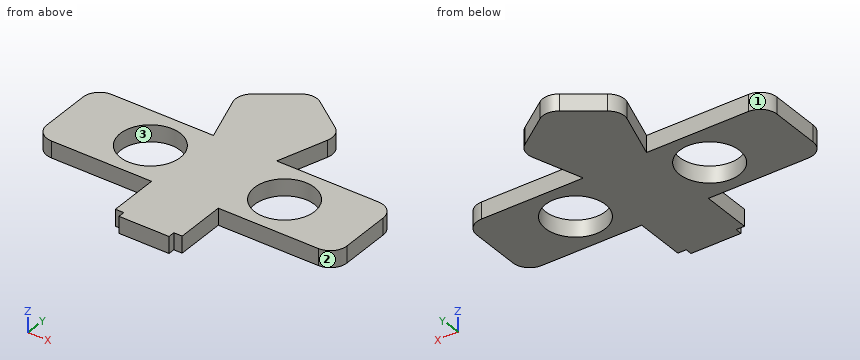
from build123d import *

# Parameters (mm, degrees)
F0_R     = 9
F0_W     = 15
F0_H     = 2
F1_DEPTH = 5


with BuildPart() as f1:
    # F0 (on Top) → F1 (new body)
    with BuildSketch(Plane.XY):
        with BuildLine():
            Line((-9.487151, 12.5), (-40, 12.5))
            ThreePointArc((-40, 12.5), (-43.535534, 11.035534), (-45, 7.5))
            Line((-45, 7.5), (-45, -7.5))
            ThreePointArc((-45, -7.5), (-43.535534, -11.035534), (-40, -12.5))
            Line((-40, -12.5), (-10, -12.5))
            Line((-10, -12.5), (10, -12.5))
            Line((10, -12.5), (40, -12.5))
            ThreePointArc((40, -12.5), (43.535534, -11.035534), (45, -7.5))
            Line((45, -7.5), (45, 7.5))
            ThreePointArc((45, 7.5), (43.535534, 11.035534), (40, 12.5))
            Line((40, 12.5), (9.487151, 12.5))
            Line((9.487151, 12.5), (-9.487151, 12.5))
        make_face()
        with Locations((-19.38206, 0)):
            Circle(F0_R, mode=Mode.SUBTRACT)
        with Locations((20.852027, 0)):
            Circle(F0_R, mode=Mode.SUBTRACT)
        with BuildLine():
            Line((-14.227962, 27.090718), (-9.487151, 12.5))
            Line((-9.487151, 12.5), (9.487151, 12.5))
            Line((9.487151, 12.5), (14.227962, 27.090718))
            ThreePointArc((14.227962, 27.090718), (14.227962, 30.180888), (12.411606, 32.680888))
            Line((12.411606, 32.680888), (2.938926, 39.563193))
            ThreePointArc((2.938926, 39.563193), (0, 40.518108), (-2.938926, 39.563193))
            Line((-2.938926, 39.563193), (-12.411606, 32.680888))
            ThreePointArc((-12.411606, 32.680888), (-14.227962, 30.180888), (-14.227962, 27.090718))
        make_face()
        Polygon((10, -12.5), (-10, -12.5), (-10, -27.5), (-7.5, -27.5), (7.5, -27.5), (10, -27.5), align=None)
        with Locations((0, -28.5)):
            Rectangle(F0_W, F0_H)
    extrude(amount=F1_DEPTH)


solid = f1.part
The model under review builds one solid part; all positions refer to its coordinate system, in mm. Face numbers are marked on the shaded views. Coordinates: 2 decimals unless noted, no trailing zeros. Write each loop counter-clockwise with the first axis right and the second up, starting at its lowest first coordinate (ties: lowest second). Pieces come first, ordered by that corner, then holes. Notation, with made-up numbers: (-27.75, 71.5) - (0.25, 71.5) arc R23 ccw to (0.25, 92.5) - close; hole circle Ø5 at (-30.75, 39). An arc over 180 degrees is marked (long way). Answer as CSV lines item,"result".
(1) We need section A-A (y = 0). Give the boundary of the cut face in (x, z), plus the area to 3 significant figures.
Data:
outline,"(-45, 0) - (-28.38, 0) - (-28.38, 5) - (-45, 5) - close; (-10.38, 0) - (11.85, 0) - (11.85, 5) - (-10.38, 5) - close; (29.85, 0) - (45, 0) - (45, 5) - (29.85, 5) - close"
area,"270 mm2"
(2) We need section B-B (z = 4.1). Give the boundary of the cut face in (x, y), plus the area to 3 significant figures.
Data:
outline,"(-45, -7.5) arc R5 ccw to (-40, -12.5) - (-10, -12.5) - (-10, -27.5) - (-7.5, -27.5) - (-7.5, -29.5) - (7.5, -29.5) - (7.5, -27.5) - (10, -27.5) - (10, -12.5) - (40, -12.5) arc R5 ccw to (45, -7.5) - (45, 7.5) arc R5 ccw to (40, 12.5) - (9.49, 12.5) - (14.23, 27.09) arc R5 ccw to (12.41, 32.68) - (2.94, 39.56) arc R5 ccw to (-2.94, 39.56) - (-12.41, 32.68) arc R5 ccw to (-14.23, 27.09) - (-9.49, 12.5) - (-40, 12.5) arc R5 ccw to (-45, 7.5) - close; hole circle Ø18 at (-19.38, 0); hole circle Ø18 at (20.85, 0)"
area,"2,660 mm2"
(3) Mouldability with a two-part tool opening along X and no side actions: class the marked faces 1, 2 and 3 as pulls with the +X half, pulls with the -X half, needs draft (parallel to the pull), parting line crosses it, or undercut.
Data:
face 1,"pulls with the -X half"
face 2,"pulls with the +X half"
face 3,"undercut"
(4) Clearance check with flat-ended pins moving along their axes: pin 1 Ø11 at (x, y) = (20.85, 0) entering from +Z; pin 2 Ø1.5 at (x, z) = (18.5, 3) entering from -Y; pin 3 Ø1 at (x, z) = (31.5, 3.5) entering from +Y; pin 4 Ø3 at (y, z) = (31, 0.5) entering from +X. State where each tip first meets the part, or that it passes through.
Data:
pin 1,"passes through"
pin 2,"stops at y = -12.5"
pin 3,"stops at y = 12.5"
pin 4,"stops at x = 14.4"
(5) We need section C-C (x = -27). Give the boundary of the cut face in (y, z), plus the area to 3 significant figures.
Data:
outline,"(-12.5, 0) - (-4.79, 0) - (-4.79, 5) - (-12.5, 5) - close; (4.79, 0) - (12.5, 0) - (12.5, 5) - (4.79, 5) - close"
area,"77.1 mm2"
(6) For line 1 along X through (y, z) = (0.5, 0.35); line 2 along X through (y, z) = (-4, 3.05); line 3 along Y through (x, z) = (40, 2.8), list the stretches that pass through material, from the lowest coordinate up. Write a range as [from, to].
Data:
line 1,"x = [-45, -28.37], [-10.4, 11.87], [29.84, 45]"
line 2,"x = [-45, -27.44], [-11.32, 12.79], [28.91, 45]"
line 3,"y = [-12.5, 12.5]"
(7) We need section D-D (y = 10.5). Give the boundary of the cut face in (x, z).
Data:
outline,"(-44, 0) - (44, 0) - (44, 5) - (-44, 5) - close"
